Part model, mm, in its own coordinate system. A direction names the side the tool comes from. Coordinates: 2 decimals unless noted, no trailing zeros. Write each loop counter-clockwise with the first axis right and the second up, starting at its lowest first coordinate (ties: lowest second). Pieces come first, ordered by that corner, then holes. Notation, with made-up numbers: (72.5, -6) - (126.5, -6) arc R27 ccw to (126.5, 21) - close; hole circle Ø3 at (64, 84.25). An arc over 180 degrees is marked (long way). Write each question's results on one line, items separated by ' | '.
Autodesk Inventor part; units mm, degrees
ref_plane "Płaszczyzna konstrukcyjna1" through (-4.8101, 8.1046, 0) normal (-1, 0, 0) x (0, 0, 1)
ref_plane "YZ Plane" through (0, 0, 0) normal (1, 0, 0) x (0, 1, 0)
ref_plane "XZ Plane" through (0, 0, 0) normal (0, 1, 0) x (-1, 0, 0)
sketch "Szkic1" plane through (0, 0, 0) normal (0, 0, 1) x (1, 0, 0)
  line L0 (-10.8101, 8.1046) -> (-12.3101, 8.1046)
  line L1 (-12.3101, 8.1046) -> (-12.3101, 11.6046)
  line L2 (-12.3101, 11.6046) -> (-10.8101, 11.6046)
  line L3 (-10.8101, 11.6046) -> (-10.8101, 8.1046)
  line L4 (-10.8101, 11.6046) -> (1.1899, 11.6046)
  line L5 (1.1899, 11.6046) -> (1.1899, 11.1716)
  line L6 (1.1899, 11.1716) -> (-10.8101, 11.1716)
  line L7 (-10.8101, 11.1716) -> (-10.8101, 11.6046)
  line L8 (1.1899, 11.6046) -> (2.6899, 11.6046)
  line L9 (2.6899, 11.6046) -> (2.6899, 8.1046)
  line L10 (2.6899, 8.1046) -> (1.1899, 8.1046)
  line L11 (1.1899, 8.1046) -> (1.1899, 11.6046)
  point P0 (0, 0)
  dimension "d0" = 1.5
  dimension "d1" = 1.5
  dimension "d2" = 15
  dimension "d3" = 0.433
  dimension "d6" = 3.5
extrude "Wyciągnięcie proste1" add sketch "Szkic1" along normal blind 13
sketch "Szkic2" plane through (-12.3101, 8.1046, 0) normal (-1, 0, 0) x (0, 0, 1)
  line L0 (0, 0) -> (13, 0)
  line L1 (13, 0) -> (7, 3.5)
  line L2 (0, 3.5) -> (13, 3.5)
  line L3 (0, 3.5) -> (0, 0)
  line L4 (13, 3.5) -> (13, 0)
  line L5 (13, 0) -> (13, 3.5)
  point P0 (0, -8.1046)
  dimension "d7" = 7
extrude "Wyciągnięcie proste2" cut sketch "Szkic2" against normal through all contours L1 L2 L4
sketch "Szkic4" plane through (-12.3101, 8.1046, 0) normal (0, -1, 0) x (1, 0, 0)
  circle A0 centre (14.25, 3) radius 0.475
  line L0 (13.5, 0) -> (13.5, 13)
  line L1 (13.5, 0) -> (15, 0)
  circle A1 centre (0.75, 3) radius 0.475
  line L2 (0, 0) -> (1.5, 0)
  line L3 (0, 0) -> (0, 13)
  point P0 (12.3101, 0)
  dimension "d10" = 0.95
  dimension "d11" = 0.75
  dimension "d12" = 3
  dimension "d13" = 3
  dimension "d14" = 0.75
  dimension "d15" = 0.95
extrude "Wyciągnięcie proste3" add sketch "Szkic4" along normal blind 1
sketch "Szkic5" plane through (-12.3101, 8.1046, 0) normal (-1, 0, 0) x (0, 0, 1)
  line L0 (0, 0) -> (13, 0)
  line L1 (0, 3.5) -> (7, 3.5)
  line L2 (13, 0) -> (7, 3.5)
  line L3 (0, 3.5) -> (7, 3.5)
  line L4 (0, 3.5) -> (0, 0)
  line L5 (0, 0) -> (13, 0)
  line L6 (6.8648, 3) -> (11.1505, 0.5)
  line L7 (0.5, 0.5) -> (0.5, 3)
  line L8 (0.5, 3) -> (6.8648, 3)
  line L9 (11.1505, 0.5) -> (12.0077, 0)
  line L10 (0.5, 0.5) -> (0.5, 0)
  line L11 (2.5, 0) -> (2.5, 3)
  line L12 (3.5, 0) -> (3.5, 3)
  point P0 (0, -8.1046)
  dimension "d19" = 0.5
  dimension "d20" = 1
  dimension "d21" = 2
extrude "Wyciągnięcie proste4" cut sketch "Szkic5" against normal blind 15 contours L10 L7 L8 L11 L0 | L12 L8 L6 L9 L0
sketch "Szkic7" plane through (0, 0, 0) normal (0, 0, -1) x (-1, 0, 0)
  line L0 (12.3101, 11.6046) -> (12.3101, 8.1046)
  line L1 (12.3101, 8.1046) -> (10.8101, 8.9706)
  line L2 (10.8101, 8.1046) -> (10.8101, 11.1046)
  line L3 (12.3101, 8.6046) -> (10.8101, 9.4706)
  line L4 (12.3101, 8.1046) -> (10.8101, 8.1046)
  point P0 (0, 0)
  dimension "d33" = 60
  dimension "d34" = 60
  dimension "d35" = 0
  dimension "d36" = 0.5
extrude "Wyciągnięcie proste6" add sketch "Szkic7" against normal blind 3 contours L0 L1 L2 L3
pattern_linear "Szyk prostokątny1" count 2 spacing 1 along (0, 1, 0) of "Wyciągnięcie proste6"
ref_plane "Płaszczyzna konstrukcyjna1" through (-4.8101, 8.1046, 0) normal (-1, 0, 0) x (0, 0, 1)
mirror "Odbij1" about plane through (-4.8101, 8.1046, 0) normal (-1, 0, 0) of "Wyciągnięcie proste6", "Szyk prostokątny1"
fillet "Zaokrąglenie1" radius 1 3 edges at (-12.3101, 11.6046, 3.5) (-4.8101, 11.6046, 7) (2.6899, 11.6046, 3.5)
properties part number "dach" material "Tworzywo sztuczne ABS"
(1) 3-axis set-ups, long thin cutter, end or side, ignore diameter. For faces 1 (the flat face through (2.1, 10.5, 2.5)), 2 (the flat face through (-11.57, 9.53, 1.49)), 3 (the cylindrical face through (2.16, 7.61, 3.42)), 4 (the flat face through (2, 11.105, 1)), 5 (the flat face through (-11.57, 10.03, 1.49)): which of +Z, -Z, +X, -X, +Y, -Y reach the whole face in a straight line?
Return value:
face 1: +X | face 2: none | face 3: -Y | face 4: +X, -X | face 5: -X
(2) Two-plate mould, pull along Y, no slides. Class faces 6 (the flat face through (-11.2, 8.3, 2.5)), 7 (the flat face through (2, 7.105, 3)), 8 (the flat face through (1.929, 10.044, 1.486)): released by +Y, released by -Y, zero draft, split by the parting line, or undercut.
Return value:
face 6: zero draft | face 7: released by -Y | face 8: undercut
(3) Flat gauge pins, fed straight in: P1, Ø1.7, axis at x = -11.5, y = 10.5, coming from the +Z side; P2, Ø0.5, axis at x = -12, z = 12.5, coming from the -Y side; P3, Ø0.7, axis at x = -11.5, y = 8.5, coming from the +Z side. Where does each tip first touch, or does it go through?
Return value:
P1: stops at z = 10.35 | P2: stops at y = 8.1 | P3: stops at z = 12.92
(4) Saw through at A-A on z = 3. Write the cut outline in (x, y).
Return value:
outline: (-12.31, 8.1) - (-12.04, 8.1) - (-12.04, 7.1) - (-11.09, 7.1) - (-11.09, 8.1) - (-10.81, 8.1) - (-10.81, 11.17) - (1.19, 11.17) - (1.19, 8.1) - (1.46, 8.1) - (1.46, 7.1) - (2.41, 7.1) - (2.41, 8.1) - (2.69, 8.1) - (2.69, 10.6) arc R1 ccw to (1.69, 11.6) - (-11.31, 11.6) arc R1 ccw to (-12.31, 10.6) - close
(5) Saw through at B-B on x = -2.5. Write the cut outline in (y, z), then the cut area to 3 significant figures.
Return value:
outline: (11.17, 0) - (11.6, 0) - (11.6, 6.73) arc R1 ccw to (11.47, 7.23) - (11.17, 7.74) - close | area: 3.19 mm^2
(6) Wall check: line 1 (X direction, y = 9.1, z = 10.5); line 2 (Y direction, x = -10.25, z = 2.5); line 3 (X direction, y = 9.8, z = 2). Give the ranges that are in metal, low to high. Write a range as from..to.
Return value:
line 1: x = -12.31..-10.81, 1.19..2.69 | line 2: y = 11.17..11.6 | line 3: x = -11.97..-11.11, 1.49..2.35
